The model under review builds one solid part; all positions refer to its coordinate system, in mm. Face numbers are marked on the shaded views. A direction names the side the tool comes from. Round coordinates to 2 decimals unless told otherwise and drop trailing zeros. Write each loop counter-clockwise with the first axis right and the second up, starting at its lowest first coordinate (ties: lowest second). Pieces come first, ordered by that corner, then holes. Notation, with made-up numbers: (-25.75, -21.5) -> (11.25, -21.5) arc R29 cw to (11.25, 12.5) -> close; hole circle Ø11 at (-12.75, -20). An arc over 180 degrees is marked (long way). Answer as a JSON object with one key per item and string values. Group by question number.
1) We need section D-D, the plane x = -2.25. Write out the cut boundary in (y, z), then the cut area to 3 significant figures.
2) We need section A-A, the plane y = 0. Write out the cut boundary in (x, z).
3) To check wall thickness, follow probe 1 along X at (y, z) = (0, 6.5); probe 2 along X at (y, z) = (0, 14); probe 3 along X at (y, z) = (-2.5, 1.75). State the ranges of each line that lie inside material, in increasing order. Write a range as [from, to].
4) We need section B-B, the plane x = 0. Write out the cut boundary in (y, z).
5) Mouldability with a two-part tool opening along X and no side actions: class the marked faces 1, 2 and 3 as pulls with the +X half, pulls with the -X half, needs draft (parallel to the pull), parting line crosses it, or undercut.
6) Machinability: for the marked faces 4, 5 and 6, which of the approach directions +Z, -Z, +X, -X, +Y, -Y give a long, thin tool a straight path to every point of the face, cutting with its end or side? Answer none if there is none.
7) We need section C-C, the plane z = 2.25. Write out the cut boundary in (x, y), then the cut area to 3 significant figures.
8) Insertion check: pin 1 Ø2 at (x, z) = (3.5, 11.5) entering from +Y; pin 2 Ø1.5 at (y, z) = (1.5, 8) entering from -X; pin 3 Ø1.6 at (y, z) = (0.5, 2.5) entering from -X. Each pin has a flat end and moves straight along its axis. Give the tip position at first contact, or say it passes through.
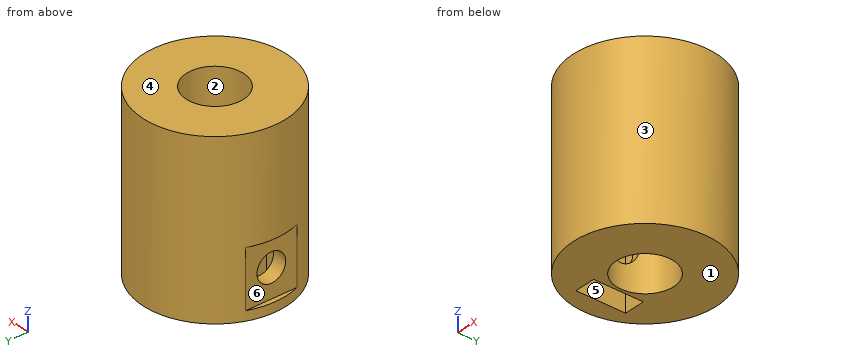
Autodesk Inventor part; units mm, degrees
ref_plane "Work Plane1" through (0, 0, 5) normal (0, 0, 1) x (1, 0, 0)
ref_plane "YZ Plane" through (0, 0, 0) normal (1, 0, 0) x (0, 1, 0)
ref_plane "XZ Plane" through (0, 0, 0) normal (0, 1, 0) x (-1, 0, 0)
sketch "Sketch1" plane through (0, 0, 0) normal (0, 0, 1) x (1, 0, 0)
  circle A0 centre (0, 0) radius 7.5
  circle A1 centre (0, 0) radius 3
  dimension "d0" = 15
  dimension "d1" = 6
extrude "Extrusion1" add sketch "Sketch1" along normal blind 17.8
ref_plane "Work Plane1" through (0, 0, 5) normal (0, 0, 1) x (1, 0, 0)
sketch "Sketch2" plane through (0, 0, 5) normal (0, 0, 1) x (1, 0, 0)
  line L0 (-5.5, -2.6) -> (-3.3, -2.6)
  line L1 (-3.3, -2.6) -> (-3.3, 2.6)
  line L2 (-3.3, 2.6) -> (-5.5, 2.6)
  line L3 (-5.5, 2.6) -> (-5.5, -2.6)
  point P0 (0, 0)
  point P1 (-5.5, 0)
  dimension "d5" = 5.5
  dimension "d6" = 2.2
  dimension "d7" = 5.2
extrude "Extrusion2" cut sketch "Sketch2" along normal mid plane 10
sketch "Sketch4" plane through (0, 0, 0) normal (1, 0, 0) x (0, 1, 0)
  circle A0 centre (0, 4) radius 1.5
  line L0 (-2.1, 0) -> (2.1, 0)
  point P0 (0, 0)
  dimension "d12" = 3
  dimension "d13" = 4
extrude "Extrusion3" cut sketch "Sketch4" against normal blind 8
sketch "Sketch5" plane through (0, 0, 0) normal (0, 1, 0) x (-1, 0, 0)
  line L0 (7.5, 0) -> (7.5, 17.8)
  line L1 (7.5, 1) -> (7, 1)
  line L2 (7, 1) -> (7, 7)
  line L3 (7, 7) -> (7.5, 7)
  line L4 (7.5, 7) -> (7.5, 1)
  line L5 (-1.5, 0) -> (9, 0)
  point P0 (0, 0)
  dimension "d16" = 6
  dimension "d17" = 7
  dimension "d18" = 0.5
extrude "Extrusion4" cut sketch "Sketch5" along normal mid plane 8
properties part number "Acople eje motor"
Here are the results:
{
 "1": {"outline": "(-7.15, 0) -> (-1.98, 0) -> (-1.98, 17.8) -> (-7.15, 17.8) -> close; (1.98, 0) -> (7.15, 0) -> (7.15, 17.8) -> (1.98, 17.8) -> close", "area": "184 mm^2"},
 "2": {"outline": "(-7.5, 0) -> (-5.5, 0) -> (-5.5, 2.5) -> (-7, 2.5) -> (-7, 1) -> (-7.5, 1) -> close; (-7.5, 7) -> (-7, 7) -> (-7, 5.5) -> (-5.5, 5.5) -> (-5.5, 10) -> (-3.3, 10) -> (-3.3, 5.5) -> (-3, 5.5) -> (-3, 17.8) -> (-7.5, 17.8) -> close; (-3.3, 0) -> (-3, 0) -> (-3, 2.5) -> (-3.3, 2.5) -> close; (3, 0) -> (7.5, 0) -> (7.5, 17.8) -> (3, 17.8) -> close"},
 "3": {"probe 1": "x = [-7, -5.5], [-3.3, -3], [3, 7.5]", "probe 2": "x = [-7.5, -3], [3, 7.5]", "probe 3": "x = [-7, -5.5], [-3.3, -1.66], [1.66, 7.07]"},
 "4": {"outline": "(-7.5, 0) -> (-3, 0) -> (-3, 17.8) -> (-7.5, 17.8) -> close; (3, 0) -> (7.5, 0) -> (7.5, 17.8) -> (3, 17.8) -> close"},
 "5": {"face 1": "needs draft", "face 2": "undercut", "face 3": "parting line crosses it"},
 "6": {"face 4": "+Z, +X, -X, +Y, -Y", "face 5": "-Z", "face 6": "-X, +Y, -Y"},
 "7": {"outline": "(-7, -2.69) arc R7.5 ccw (long way) to (-7, 2.69) -> close; hole (-5.5, -2.6) -> (-3.3, -2.6) -> (-3.3, 2.6) -> (-5.5, 2.6) -> close; hole circle Ø6 at (0, 0)", "area": "135 mm^2"},
 "8": {"pin 1": "stops at y = 7.07", "pin 2": "stops at x = -7.46", "pin 3": "stops at x = -7"}
}
